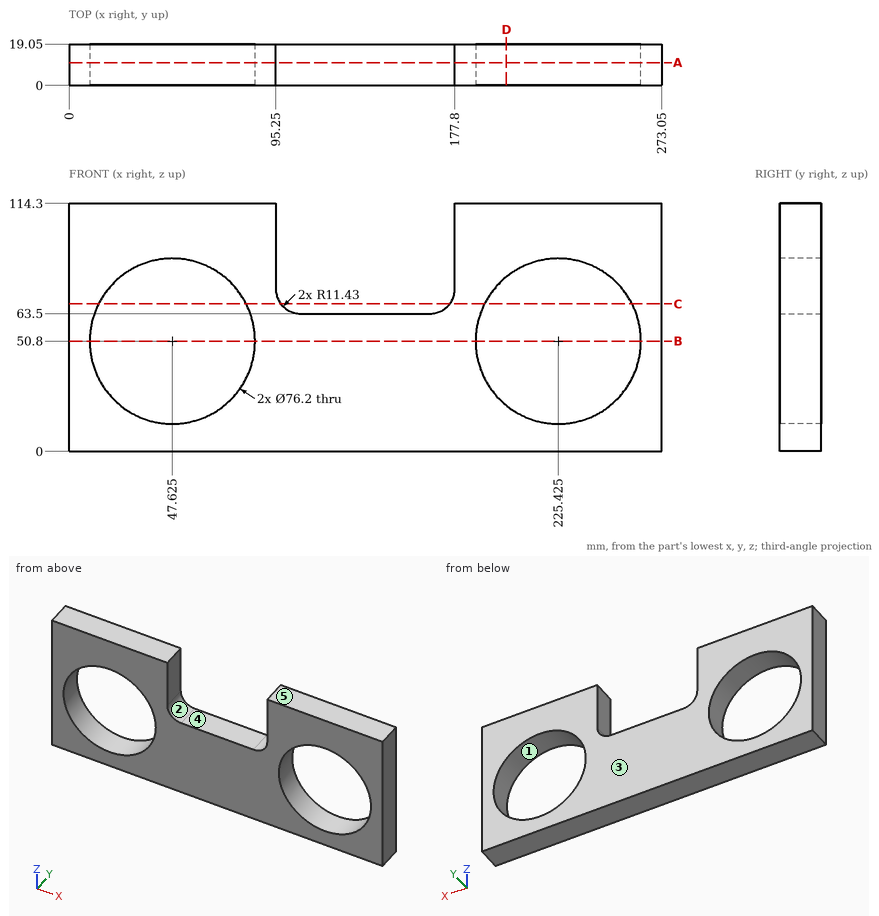
Can you work these out from the drawing? Everything is in mm from the part's minimum corner. A direction names the side the tool comes from. Give positions to 0.01 mm unless a question says otherwise; leave off trailing zeros. Order: outer loops, then holes, each group sorted by start corner. A loop starts at its lowest first (then second) coordinate and runs counter-clockwise, first axis right, second up. Notation, with made-up numbers: M 63,53 L 91,53 A16 ccw 91,80 Z; hole C -25,38 d5. An arc over 180 degrees is marked long. One line per item, written item: value.
Item 1: For pin 1 (9.5 mm diameter, centred on x = 130.5, y = 13, fed in from +Z), with a flat end and sliding along its axis, tell me the tip position at first contact or that it passes through.
Verdict:
pin 1: z = 63.5
Item 2: If we section it at B-B on z = 50.8: Write out the boundary of the cut face in (x, y) (3 decimals), and give its area (3 significant figures).
Verdict:
outline: M 0,0 L 9.525,0 L 9.525,19.05 L 0,19.05 Z; M 85.725,0 L 187.325,0 L 187.325,19.05 L 85.725,19.05 Z; M 263.525,0 L 273.05,0 L 273.05,19.05 L 263.525,19.05 Z
area: 2,300 mm2
Item 3: If we section it at C-C on z = 68: Write out the boundary of the cut face in (x, y).
Verdict:
outline: M 0,0 L 13.63,0 L 13.63,19.05 L 0,19.05 Z; M 81.62,0 L 97.59,0 L 97.59,19.05 L 81.62,19.05 Z; M 175.46,0 L 191.43,0 L 191.43,19.05 L 175.46,19.05 Z; M 259.42,0 L 273.05,0 L 273.05,19.05 L 259.42,19.05 Z
Item 4: Please list where these lines run through material, in increasing order: line 1 (X direction, y = 12.25, z = 38.5); line 2 (X direction, y = 9, z = 98); line 3 (X direction, y = 2.25, z = 69.5).
Verdict:
line 1: 0 to 11.57, 83.68 to 189.37, 261.48 to 273.05
line 2: 0 to 95.25, 177.8 to 273.05
line 3: 0 to 14.43, 80.82 to 96.62, 176.43 to 192.23, 258.62 to 273.05
Item 5: If we section it at D-D on x = 201.5: Write out the boundary of the cut face in (y, z), and give its area (3 significant figures).
Verdict:
outline: M 0,0 L 19.05,0 L 19.05,21.15 L 0,21.15 Z; M 0,80.45 L 19.05,80.45 L 19.05,114.3 L 0,114.3 Z
area: 1,050 mm2
Item 6: If we mould it in two halves opening along Z, with no side actions, what happens to the marked faces 1, 2 and 3? For each: pulls with the +Z half, pulls with the -Z half, needs draft (parallel to the pull), parting line crosses it, or undercut.
Verdict:
face 1: undercut
face 2: pulls with the +Z half
face 3: needs draft
Item 7: If we section it at A-A on y = 10.5: Write out the boundary of the cut face in (x, z) (3 decimals).
Verdict:
outline: M 0,0 L 273.05,0 L 273.05,114.3 L 177.8,114.3 L 177.8,74.93 A11.43 cw 166.37,63.5 L 106.68,63.5 A11.43 cw 95.25,74.93 L 95.25,114.3 L 0,114.3 Z; hole C 47.625,50.8 d76.2; hole C 225.425,50.8 d76.2
Item 8: For the marked faces 4 and 5, which set-ups out of +Z, -Z, +X, -X, +Y, -Y let a thin tool reach every point of the face, with its end or its side?
Verdict:
face 4: +Z, +Y, -Y
face 5: +Z, +X, -X, +Y, -Y
